Read the model definition and answer for the solid it produces. Units are mm, in the model's axes. A direction names the side the tool comes from. Round coordinates to 2 decimals unless told otherwise and drop trailing zeros. Write each loop counter-clockwise with the first axis right and the second up, starting at its lowest first coordinate (ties: lowest second). Pieces come first, ordered by that corner, then holes. Notation, with made-up numbers: (-20.5, 40) -> (35.5, 40) arc R21 ccw to (35.5, 58) -> close; hole circle Ø6 at (43.25, 50.25). An arc over 180 degrees is marked (long way). Return JSON: item names as keys, results as strings.
from build123d import *

# Parameters (mm, degrees)
SKETCH1_R           = 5
BOSS_EXTRUDE1_DEPTH = 13
SKETCH2_R           = 7.5
BOSS_EXTRUDE2_DEPTH = 8
SKETCH3_R           = 7.5
BOSS_EXTRUDE3_DEPTH = 7
SKETCH4_R           = 5
BOSS_EXTRUDE4_DEPTH = 13
SKETCH5_R           = 5
CUT_EXTRUDE1_DEPTH  = 43.558312936
SKETCH6_R           = 17.5
BOSS_EXTRUDE5_DEPTH = 1
SKETCH7_R           = 5
CUT_EXTRUDE2_DEPTH  = 27.009613607


with BuildPart() as part:
    # Sketch1 → Boss-Extrude1 (new body)
    with BuildSketch(Plane(origin=(0, 0, 0), x_dir=(1, 0, 0), z_dir=(0, 1, 0))):
        with Locations(Location((0, 0, 0), (0, 0, 90))):
            Circle(SKETCH1_R)
    extrude(amount=BOSS_EXTRUDE1_DEPTH)

    # Sketch2 → Boss-Extrude2 (add)
    with BuildSketch(Plane(origin=(0, 13, 0), x_dir=(1, 0, 0), z_dir=(0, 1, 0))):
        with Locations(Location((0, -1.1, 0), (0, 0, 270))):
            Circle(SKETCH2_R)
    extrude(amount=BOSS_EXTRUDE2_DEPTH)

    # Sketch3 → Boss-Extrude3 (add)
    with BuildSketch(Plane(origin=(0, 21, 0), x_dir=(1, 0, 0), z_dir=(0, 1, 0))):
        with Locations(Location((0, 1.1, 0), (0, 0, 188.433804098))):
            Circle(SKETCH3_R)
    extrude(amount=BOSS_EXTRUDE3_DEPTH)

    # Sketch4 → Boss-Extrude4 (add)
    with BuildSketch(Plane(origin=(0, 28, 0), x_dir=(1, 0, 0), z_dir=(0, 1, 0))):
        with Locations(Location((0, 0, 0), (0, 0, 90))):
            Circle(SKETCH4_R)
    extrude(amount=BOSS_EXTRUDE4_DEPTH)

    # Sketch5 → Cut-Extrude1 (cut, through all)
    with BuildSketch(Plane.XZ):
        with Locations(Location((0, 0, 0), (0, 0, 90))):
            Circle(SKETCH5_R)
    extrude(amount=-CUT_EXTRUDE1_DEPTH, mode=Mode.SUBTRACT)

    # Sketch6 → Boss-Extrude5 (add)
    with BuildSketch(Plane.XZ.offset(-21)):
        with Locations(Location((0, 0, 0), (0, 0, 270))):
            Circle(SKETCH6_R)
    extrude(amount=BOSS_EXTRUDE5_DEPTH)

    # Sketch7 → Cut-Extrude2 (cut, through all)
    with BuildSketch(Plane(origin=(0, 21, 0), x_dir=(1, 0, 0), z_dir=(0, 1, 0))):
        with Locations(Location((0, 0, 0), (0, 0, 270))):
            Circle(SKETCH7_R)
    extrude(amount=-CUT_EXTRUDE2_DEPTH, mode=Mode.SUBTRACT)


solid = part.part
Item 1: A tool of negligible diameter and unlimited length cuts with its end or side. For faces 1 (the cylindrical face through (-2.87, 16.45, 8.03)), 2 (the flat face through (-8, 21, 0)), 3 (the flat face through (-4, 28, -4)), from which of +Z, -Z, +X, -X, +Y, -Y can it reach the whole face along a straight path? Write none if from no direction.
Worked answers:
{"face 1": "-Y", "face 2": "+Y", "face 3": "+Z, -Z, +X, -X, +Y"}
Item 2: Section B-B (z = 4.5) is taken. Give the vertices of the cut face in (x, y).
Worked answers:
{"outline": "(-16.91, 20) -> (-6.69, 20) -> (-6.69, 13) -> (-2.18, 13) -> (-2.18, 28) -> (-4.99, 28) -> (-4.99, 21) -> (-16.91, 21) -> close; (2.18, 13) -> (6.69, 13) -> (6.69, 20) -> (16.91, 20) -> (16.91, 21) -> (4.99, 21) -> (4.99, 28) -> (2.18, 28) -> close"}
Item 3: Straight lines are drawn through the part: L1, parallel to Y at x = -8, z = 3.5; L2, parallel to X at y = 17.25, z = 0; L3, parallel to Z at x = 1, y = 26.25. For each, find the intervals that lie inside material, in ascending order. Write a range as [from, to].
Worked answers:
{"L1": "y = [20, 21]", "L2": "x = [-7.42, -5], [5, 7.42]", "L3": "z = [-8.53, -4.9], [4.9, 6.33]"}
Item 4: For a pull along X with two mould halves and no side action, classify faces 4 (the cylindrical face through (4.88, 20.4, -1.08)), 5 (the flat face through (0, 20, -8)), 6 (the cylindrical face through (7.46, 24.45, -1.87)) as released by +X, released by -X, zero draft, split by the parting line, or undercut.
Worked answers:
{"face 4": "undercut", "face 5": "zero draft", "face 6": "split by the parting line"}
Item 5: Flat-ended cylindrical pins translate along their axes: pin 1 (6 mm diameter, centred on x = -4, y = 26, fed in from -Z); pin 2 (8 mm diameter, centred on x = -9.5, y = 21.5, fed in from -Z); pin 3 (5 mm diameter, centred on y = 20.5, z = 9.5, fed in from +X). Find the tip coordinate at first contact, or state that the pin passes through.
Worked answers:
{"pin 1": "stops at z = -8.53", "pin 2": "stops at z = -16.6", "pin 3": "stops at x = 16.04"}
Item 6: Section A-A (x = 0) is taken. Give the vertices of the cut face in (y, z), then the cut area to 3 significant figures.
Worked answers:
{"outline": "(13, -6.4) -> (20, -6.4) -> (20, -17.5) -> (21, -17.5) -> (21, -8.6) -> (28, -8.6) -> (28, -5) -> (13, -5) -> close; (13, 5) -> (28, 5) -> (28, 6.4) -> (21, 6.4) -> (21, 17.5) -> (20, 17.5) -> (20, 8.6) -> (13, 8.6) -> close", "area": "95.0 mm2"}
Item 7: Section D-D (z = -15) is taken. Give the vertices of the cut face in (x, y), then the cut area to 3 significant figures.
Worked answers:
{"outline": "(-9.01, 20) -> (9.01, 20) -> (9.01, 21) -> (-9.01, 21) -> close", "area": "18.0 mm2"}
Item 8: Section C-C (y = 14.5) is taken. Give the vertices of the cut face in (x, z), then the cut area to 3 significant figures.
Worked answers:
{"outline": "circle Ø15 at (0, 1.1); hole circle Ø10 at (0, 0)", "area": "98.2 mm2"}
